Design review of the part built by this model. Coordinates are the model's own, in mm. A direction names the side the tool comes from. Give positions to 0.01 mm unless a question says otherwise; leave off trailing zeros. Order: outer loops, then holes, each group sorted by start corner. A loop starts at its lowest first (then second) coordinate and runs counter-clockwise, first axis right, second up. Notation, with made-up numbers: (80.5, -21) -> (122.5, -21) arc R12 ccw to (122.5, -8) -> close; hole circle Ø11 at (42.25, 50). An arc over 180 degrees is marked (long way). Return JSON: item names as keys, results as strings.
```python
from build123d import *

# Parameters (mm, degrees)
BOSS_EXTRUDE1_DEPTH     = 9.525
BOSS_EXTRUDE2_DEPTH     = 25.4
SKETCH4_W               = 63.5
SKETCH4_H               = 3.175
CUT_EXTRUDE1_DEPTH      = 6.35
CUT_EXTRUDE2_DEPTH      = 45.095938092
CUT_EXTRUDE2_DEPTH_BACK = 45.095938092
SKETCH5_W               = 50.8
SKETCH5_H               = 1.5875


with BuildPart() as part:
    # Sketch1 → Boss-Extrude1 (new body)
    with BuildSketch(Plane.XY):
        Polygon((-29.21, -11.1125), (29.21, -11.1125), (29.21, -6.0325), (34.29, -6.0325), (34.29, 6.0325), (29.21, 6.0325), (29.21, 11.1125), (-29.21, 11.1125), (-29.21, 6.0325), (-34.29, 6.0325), (-34.29, -6.0325), (-29.21, -6.0325), align=None)
    extrude(amount=BOSS_EXTRUDE1_DEPTH)

    # Sketch3 → Boss-Extrude2 (add)
    with BuildSketch(Plane.XY.offset(9.525)):
        Polygon((-29.21, 11.1125), (-25.4, 11.1125), (-25.4, 1.5875), (-31.75, 1.5875), (-31.75, -1.5875), (-25.4, -1.5875), (-25.4, -11.1125), (-29.21, -11.1125), (-29.21, -6.0325), (-34.29, -6.0325), (-34.29, 6.0325), (-29.21, 6.0325), align=None)
        Polygon((25.4, -1.5875), (25.4, -11.1125), (29.21, -11.1125), (29.21, -6.0325), (34.29, -6.0325), (34.29, 6.0325), (29.21, 6.0325), (29.21, 11.1125), (25.4, 11.1125), (25.4, 1.5875), (31.75, 1.5875), (31.75, -1.5875), align=None)
    extrude(amount=BOSS_EXTRUDE2_DEPTH)

    # Sketch4 → Cut-Extrude1 (cut)
    with BuildSketch(Plane.XY.offset(9.525)):
        Rectangle(SKETCH4_W, SKETCH4_H)
    extrude(amount=-CUT_EXTRUDE1_DEPTH, mode=Mode.SUBTRACT)

    # Sketch5 → Cut-Extrude2 (cut, two sides: drawn at the far end of the back side and taken through both)
    with BuildSketch(Plane.XY.offset(9.525).offset(-CUT_EXTRUDE2_DEPTH_BACK)):
        with Locations((0, 10.31875)):
            Rectangle(SKETCH5_W, SKETCH5_H)
        with Locations((0, -10.31875)):
            Rectangle(SKETCH5_W, SKETCH5_H)
    extrude(amount=CUT_EXTRUDE2_DEPTH + CUT_EXTRUDE2_DEPTH_BACK, mode=Mode.SUBTRACT)


solid = part.part
```
Item 1: For pin 1 (1.5 mm diameter, centred on y = 7.5, z = 22, fed in from -X); pin 2 (1.5 mm diameter, centred on x = -31, z = 25.5, fed in from -Y); pin 3 (5 mm diameter, centred on y = -7.5, z = 16, fed in from -X); pin 4 (2.5 mm diameter, centred on x = -7.5, y = -6.5, fed in from +Z) (3 decimals), all flat-tipped, find the tip position at first contact; note any pin that passes through.
Result set:
{"pin 1": "stops at x = -29.21", "pin 2": "stops at y = -6.03", "pin 3": "stops at x = -34.29", "pin 4": "stops at z = 9.525"}
Item 2: Add section B-B (x = 2). Give the boundary of the cut face in (y, z) (1 decimal).
Result set:
{"outline": "(-9.5, 0) -> (9.5, 0) -> (9.5, 9.5) -> (1.6, 9.5) -> (1.6, 3.2) -> (-1.6, 3.2) -> (-1.6, 9.5) -> (-9.5, 9.5) -> close"}
Item 3: Mouldability with a two-part tool opening along Y and no side actions: class faces 6 (the face through (-27, 11.112, 17)), 7 (the face through (-31.75, 0, 19)), 8 (the face through (-29.21, -9, 17)) as released by +Y, released by -Y, zero draft, split by the parting line, or undercut.
Result set:
{"face 6": "released by +Y", "face 7": "undercut", "face 8": "zero draft"}
Item 4: Add section A-A (y = 3.5). Give the boundary of the cut face in (x, z) (3 decimals).
Result set:
{"outline": "(-34.29, 0) -> (34.29, 0) -> (34.29, 34.925) -> (25.4, 34.925) -> (25.4, 9.525) -> (-25.4, 9.525) -> (-25.4, 34.925) -> (-34.29, 34.925) -> close"}
Item 5: Wall thickness on L1, parallel to Y at x = 7, z = 6 (1 decimal); L2, parallel to Y at x = -31, z = 9.5; L3, parallel to X at y = 4.5, z = 27.5: over which ranges is each line inside the solid? List them lowest first. Write a range as [from, to].
Result set:
{"L1": "y = [-9.5, -1.6], [1.6, 9.5]", "L2": "y = [-6.03, -1.59], [1.59, 6.03]", "L3": "x = [-34.29, -25.4], [25.4, 34.29]"}
Item 6: Machinability: for faces 1 (the face through (0, -6, 9.525)), 2 (the face through (0, -9.525, 5)), 3 (the face through (0, -1.588, 8)), 4 (the face through (29.21, -9, 17)), 5 (the face through (29.21, 9, 17)), which of the approach directions +Z, -Z, +X, -X, +Y, -Y give a long, thin tool a straight path to every point of the face, cutting with its end or side? Answer none if there is none.
Result set:
{"face 1": "+Z, +Y, -Y", "face 2": "+Z, -Z, -Y", "face 3": "+Z", "face 4": "+Z, -Z, +X, -Y", "face 5": "+Z, -Z, +X, +Y"}
